from build123d import *

# Parameters (mm, degrees)
F1_DEPTH = 7
F2_R     = 2.125
F3_DEPTH = 10
F4_R     = 1
F5_DEPTH = 1


# Not quite as in the source:
# - a feature names something its author has since deleted; it is built from what else it names


with BuildPart() as f1:
    # F0 (on Top) → F1 (new body)
    with BuildSketch(Plane.XY):
        with BuildLine():
            ThreePointArc((-23.401635828, 2.1478921234), (-23.2315061267, 3.5421918479), (-22.9783775489, 4.9238364331))
            Line((-22.9783775489, 4.9238364331), (-32.5732277849, 4.9238364331))
            Line((-32.5732277849, 4.9238364331), (-32.5732277849, 2.1478921234))
            Line((-32.5732277849, 2.1478921234), (-23.401635828, 2.1478921234))
        make_face()
        with BuildLine():
            Line((-32.5732277849, -5.0761635669), (-22.9452078535, -5.0761635669))
            ThreePointArc((-22.9452078535, -5.0761635669), (-23.2124017724, -3.6652972535), (-23.3929275249, -2.2407458164))
            Line((-23.3929275249, -2.2407458164), (-32.5732277849, -2.2407458164))
            Line((-32.5732277849, -2.2407458164), (-32.5732277849, -5.0761635669))
        make_face()
        with BuildLine():
            ThreePointArc((-22.9452078535, -5.0761635669), (2.55319559, -23.3608902287), (23.5, 0))
            ThreePointArc((23.5, 0), (2.4756946097, 23.3692305436), (-22.9783775489, 4.9238364331))
            Line((-22.9783775489, 4.9238364331), (-17.5732277849, 4.9238364331))
            ThreePointArc((-17.5732277849, 4.9238364331), (2.4850646798, 18.080015308), (18.25, 0))
            ThreePointArc((18.25, 0), (2.4850646798, -18.080015308), (-17.5732277849, -4.9238364331))
            Line((-17.5732277849, -4.9238364331), (-17.5732277849, -5.0761635669))
            Line((-17.5732277849, -5.0761635669), (-22.9452078535, -5.0761635669))
        make_face()
        with BuildLine():
            Line((-17.5732277849, 4.9238364331), (-22.9783775489, 4.9238364331))
            ThreePointArc((-22.9783775489, 4.9238364331), (-23.2315061267, 3.5421918479), (-23.401635828, 2.1478921234))
            Line((-23.401635828, 2.1478921234), (-18.1231636153, 2.1478921234))
            ThreePointArc((-18.1231636153, 2.1478921234), (-17.9020824613, 3.5465396584), (-17.5732277849, 4.9238364331))
        make_face()
        with BuildLine():
            ThreePointArc((-23.3929275249, -2.2407458164), (-23.2124017724, -3.6652972535), (-22.9452078535, -5.0761635669))
            Line((-22.9452078535, -5.0761635669), (-17.5732277849, -5.0761635669))
            Line((-17.5732277849, -5.0761635669), (-17.5732277849, -4.9238364331))
            ThreePointArc((-17.5732277849, -4.9238364331), (-17.9020824613, -3.5465396584), (-18.1231636153, -2.1478921234))
            Line((-18.1231636153, -2.1478921234), (-18.1231636153, -2.2407458164))
            Line((-18.1231636153, -2.2407458164), (-23.3929275249, -2.2407458164))
        make_face()
    extrude(amount=F1_DEPTH)

    # F2 (on face) → F3 (cut)
    with BuildSketch(Plane.XZ.offset(5.0761635669)):
        with Locations((-27.5732277849, 3.5)):
            Circle(F2_R)
    extrude(amount=-F3_DEPTH, mode=Mode.SUBTRACT)

    # F4 (on face) → F5 (join, symmetric)
    with BuildSketch(Plane.XY.offset(7)):
        with Locations((0, -20.875)):
            Circle(F4_R)
        with Locations((0, 20.875)):
            Circle(F4_R)
    extrude(amount=F5_DEPTH, both=True)


solid = f1.part
Model file for the job. Use its own axes, mm. A direction names the side the tool comes from. Round coordinates to 2 decimals unless told otherwise and drop trailing zeros. Loops run counter-clockwise (first coordinate to the right, second up) from the corner with the lowest first, then second, coordinate; pieces in that order, holes last.
1. Band-saw the part on B-B, the plane z = 2.75. List the corners of the cut face in (x, y), and give its area (3 significant figures).
Check values:
outline: (-32.57, -5.08) - (-29.56, -5.08) - (-29.56, -2.24) - (-32.57, -2.24) - close; (-32.57, 2.15) - (-29.56, 2.15) - (-29.56, 4.92) - (-32.57, 4.92) - close; (-25.58, -5.08) - (-22.95, -5.08) arc R23.5 ccw (long way) to (-22.98, 4.92) - (-25.58, 4.92) - (-25.58, 2.15) - (-18.12, 2.15) arc R18.25 cw (long way) to (-18.12, -2.15) - (-18.12, -2.24) - (-25.58, -2.24) - close
area: 696 mm2
2. Tool access for faces 4 (the flat face through (-25, -2.241, 3)), 5 (the cylindrical face through (-0.22, 19.9, 7.51)), 6 (the flat face through (-30, -5.076, 3)): list every direction of +Z, -Z, +X, -X, +Y, -Y with a clear straight run to the whole face (end or side of a thin tool).
Check values:
face 4: +Z, -Z, -X
face 5: +Z
face 6: +Z, -Z, -X, -Y
3. Mould opens along Y. For faces 1 (the cylindrical face through (-26.593, -3.678, 1.615)), 2 (the flat face through (-30, 4.924, 3)), 3 (the flat face through (-25, 2.148, 3)) say: +Y half, -Y half, draft (parallel to the pull), parting line (faces both ways), or undercut.
Check values:
face 1: draft
face 2: +Y half
face 3: undercut
4. Band-saw the part on D-D, the plane x = -19. List the corners of the cut face in (y, z), and give its area (3 significant figures).
Check values:
outline: (-13.83, 0) - (-2.24, 0) - (-2.24, 7) - (-13.83, 7) - close; (2.15, 0) - (13.83, 0) - (13.83, 7) - (2.15, 7) - close
area: 163 mm2
5. Wall check: probe 1 along Y at (x, z) = (-0.5, 4.25); probe 2 along X at (y, z) = (3, 4.75); probe 3 along Y at (x, z) = (-14, 2.75). Give the ranges that are in metal, low to high.
Check values:
probe 1: y = -23.49 to -18.24, 18.24 to 23.49
probe 2: x = -32.57 to -29.29, -25.85 to -18, 18 to 23.31
probe 3: y = -18.87 to -11.71, 11.71 to 18.87
6. Band-saw the part on C-C, the plane y = 14. List the corners of the cut face in (x, z), and give its area (3 significant figures).
Check values:
outline: (-18.87, 0) - (-11.71, 0) - (-11.71, 7) - (-18.87, 7) - close; (11.71, 0) - (18.87, 0) - (18.87, 7) - (11.71, 7) - close
area: 100 mm2
7. Drop flat-ended pins along their axis: P1, Ø3.5, axis at x = -29, z = 3, coming from the -Y side; P2, Ø4, axis at x = 17, y = -18.5, coming from the +Z side; P3, Ø3.5, axis at x = -25.5, z = 2.5, coming from the +Y side. Give the stop position or say it passes through.
Check values:
P1: stops at y = -5.08
P2: stops at z = 7
P3: stops at y = 4.92
8. Band-saw the part on A-A, the plane x = 0. List the corners of the cut face in (y, z) (3 decimals), and give its area (3 significant figures).
Check values:
outline: (-23.5, 0) - (-18.25, 0) - (-18.25, 7) - (-19.875, 7) - (-19.875, 8) - (-21.875, 8) - (-21.875, 7) - (-23.5, 7) - close; (18.25, 0) - (23.5, 0) - (23.5, 7) - (21.875, 7) - (21.875, 8) - (19.875, 8) - (19.875, 7) - (18.25, 7) - close
area: 77.5 mm2
